Build history of the part. All positions in model axes, mm. Face numbers are marked on the shaded views. A direction names the side the tool comes from. Round coordinates to 2 decimals unless told otherwise and drop trailing zeros. Order: outer loops, then holes, each group sorted by start corner. A loop starts at its lowest first (then second) coordinate and runs counter-clockwise, first axis right, second up. Notation, with made-up numbers: (2, 73) -> (16, 73) arc R25 cw to (16, 91) -> close; hole circle Ø10 at (14.5, 66). An arc over 180 degrees is marked (long way). Answer as a JSON object with one key per item and string values.
from build123d import *

# Parameters (mm, degrees)
SKETCH035_W     = 11
SKETCH035_H     = 20
PAD019_DEPTH    = 2
SKETCH036_W     = 6.5
SKETCH036_H     = 6.25
POCKET012_DEPTH = 5
FILLET007_R     = 2
CHAMFER_SIZE    = 1.9
SKETCH037_W     = 1.384659
SKETCH037_H     = 1.938071
SKETCH037_W_2   = 0.88585
SKETCH037_H_2   = 2.057402
POCKET013_DEPTH = 22
FILLET008_R     = 0.5
SKETCH045_W     = 9
SKETCH045_H     = 18
SKETCH045_W_2   = 6.5
SKETCH045_H_2   = 6.25
PAD021_DEPTH    = 1.5


with BuildPart() as part:
    # Sketch035 → Pad019 (new body)
    with BuildSketch(Plane.XY):
        with Locations((0, -47)):
            Rectangle(SKETCH035_W, SKETCH035_H)
    extrude(amount=-PAD019_DEPTH)

    # Sketch036 → Pocket012 (cut)
    with BuildSketch(Plane.XY):
        with Locations((0, -42.375)):
            Rectangle(SKETCH036_W, SKETCH036_H)
        with Locations((0, -51.625)):
            Rectangle(SKETCH036_W, SKETCH036_H)
    extrude(amount=-POCKET012_DEPTH, mode=Mode.SUBTRACT)

    # Fillet007
    fillet007_edges = [part.edges().sort_by_distance(p)[0] for p in [
        (-5.5, -37, -1),
        (5.5, -37, -1),
        (5.5, -57, -1),
        (-5.5, -57, -1),
    ]]
    fillet(fillet007_edges, radius=FILLET007_R)

    # Chamfer
    chamfer_edges = [part.edges().sort_by_distance(p)[0] for p in [
        (0, -37, -2),
        (-4.914214, -37.585786, -2),
        (4.914214, -37.585786, -2),
        (5.5, -47, -2),
        (4.914214, -56.414214, -2),
        (0, -57, -2),
        (-5.5, -47, -2),
        (-4.914214, -56.414214, -2),
    ]]
    chamfer(chamfer_edges, length=CHAMFER_SIZE)

    # Sketch037 → Pocket013 (cut)
    with BuildSketch(Plane.XZ.offset(36)):
        with Locations((5.692301, -0.969035)):
            Rectangle(SKETCH037_W, SKETCH037_H)
        with Locations((-5.443283, -1.028701)):
            Rectangle(SKETCH037_W_2, SKETCH037_H_2)
    extrude(amount=POCKET013_DEPTH, mode=Mode.SUBTRACT)

    # Fillet008
    fillet008_edges = [part.edges().sort_by_distance(p)[0] for p in [
        (4.999972, -47, -0.600028),
        (-5.000358, -47, -0.599642),
        (-5.000358, -55.695597, -0.446238),
        (4.999972, -55.695848, -0.446482),
        (-5.000358, -38.304403, -0.446238),
        (4.999972, -38.304152, -0.446482),
    ]]
    fillet(fillet008_edges, radius=FILLET008_R)

    # Sketch045 → Pad021 (join)
    with BuildSketch(Plane.XY):
        with Locations((0, -47)):
            Rectangle(SKETCH045_W, SKETCH045_H)
        with Locations((0, -42.375)):
            Rectangle(SKETCH045_W_2, SKETCH045_H_2, mode=Mode.SUBTRACT)
        with Locations((0, -51.625)):
            Rectangle(SKETCH045_W_2, SKETCH045_H_2, mode=Mode.SUBTRACT)
    extrude(amount=PAD021_DEPTH)


solid = part.part
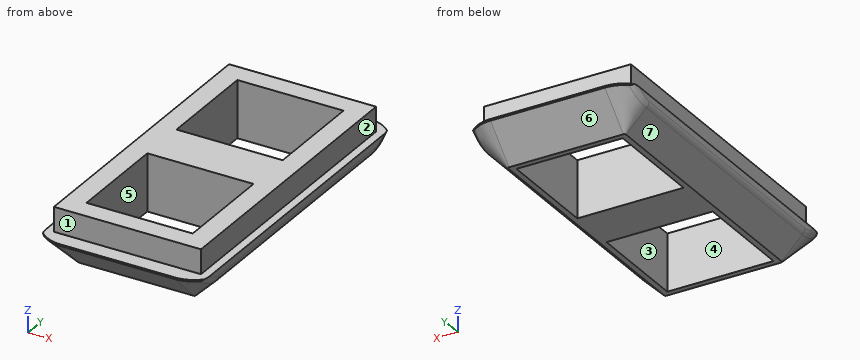
1) Flat gauge pins, fed straight in: pin 1 Ø1.5 at (x, z) = (0.5, -1.5) entering from -Y; pin 2 Ø6 at (x, y) = (1, -45) entering from -Z; pin 3 Ø1.5 at (x, z) = (2, -1) entering from -Y; pin 4 Ø1.2 at (x, z) = (0.5, 1) entering from +Y. Where does each tip first touch, or does it go through?
Checked values:
{"pin 1": "stops at y = -56.35", "pin 2": "stops at z = -2", "pin 3": "stops at y = -56.85", "pin 4": "stops at y = -38"}
2) Cut at C-C, the plane y = -54. Give the cut face in (x, z), plus the area to 3 significant figures.
Checked values:
{"outline": "(-5, -0.39) arc R0.5 ccw to (-4.85, -0.75) -> (-3.6, -2) -> (-3.25, -2) -> (-3.25, 1.5) -> (-4.5, 1.5) -> (-4.5, 0) -> (-5, 0) -> close; (3.25, -2) -> (3.6, -2) -> (4.85, -0.75) arc R0.5 ccw to (5, -0.39) -> (5, 0) -> (4.5, 0) -> (4.5, 1.5) -> (3.25, 1.5) -> close", "area": "8.78 mm²"}
3) Cut at D-D, the plane y = -47.75. Give the cut face in (x, z).
Checked values:
{"outline": "(-5, -0.39) arc R0.5 ccw to (-4.85, -0.75) -> (-3.6, -2) -> (3.6, -2) -> (4.85, -0.75) arc R0.5 ccw to (5, -0.39) -> (5, 0) -> (4.5, 0) -> (4.5, 1.5) -> (-4.5, 1.5) -> (-4.5, 0) -> (-5, 0) -> close"}
4) Pull direction Y, two halves, no side cores. Call the marked faces 4, 5, 6 and 7: pulls with the +Y half, pulls with the -Y half, needs draft (parallel to the pull), parting line crosses it, or undercut.
Checked values:
{"face 4": "undercut", "face 5": "undercut", "face 6": "pulls with the +Y half", "face 7": "needs draft"}
5) Cut at B-B, the plane z = -1. Give the cut face in (x, y).
Checked values:
{"outline": "(-4.6, -55) arc R1.1 ccw to (-3.5, -56.1) -> (3.5, -56.1) arc R1.1 ccw to (4.6, -55) -> (4.6, -39) arc R1.1 ccw to (3.5, -37.9) -> (-3.5, -37.9) arc R1.1 ccw to (-4.6, -39) -> close; hole (-3.25, -54.75) -> (3.25, -54.75) -> (3.25, -48.5) -> (-3.25, -48.5) -> close; hole (-3.25, -45.5) -> (3.25, -45.5) -> (3.25, -39.25) -> (-3.25, -39.25) -> close"}
6) Probe L1, parallel to Y at x = 1.75, z = -0.7; L2, parallel to Y at x = 1.5, z = 0.2; L3, parallel to X at y = -54, z = 0.35. List the from-to ranges inside material, lowest first. Write a range as from..to.
Checked values:
{"L1": "y = -56.4..-54.75, -48.5..-45.5, -39.25..-37.6", "L2": "y = -56..-54.75, -48.5..-45.5, -39.25..-38", "L3": "x = -4.5..-3.25, 3.25..4.5"}
7) Cut at A-A, the plane x = 1.5. Give the cut face in (y, z), plus the area to 3 significant figures.
Checked values:
{"outline": "(-57, -0.1) -> (-55.1, -2) -> (-54.75, -2) -> (-54.75, 1.5) -> (-56, 1.5) -> (-56, 0) -> (-57, 0) -> close; (-48.5, -2) -> (-45.5, -2) -> (-45.5, 1.5) -> (-48.5, 1.5) -> close; (-39.25, -2) -> (-38.9, -2) -> (-37, -0.1) -> (-37, 0) -> (-38, 0) -> (-38, 1.5) -> (-39.25, 1.5) -> close", "area": "19.6 mm²"}
8) Which spindle directions (+Z, -Z, +X, -X, +Y, -Y) get a long thin tool onto all of the face, cutting with end or side? Do the marked faces 1, 2 and 3. Say none if no direction does.
Checked values:
{"face 1": "+Z, +X, -X, -Y", "face 2": "+Z, +X, +Y, -Y", "face 3": "+Z, -Z"}
